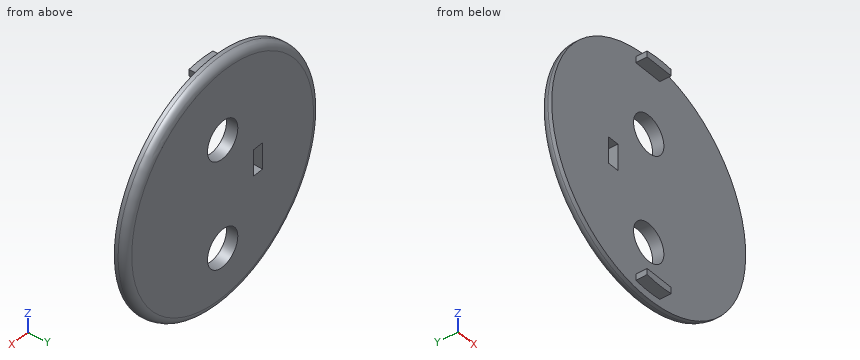
```python
from build123d import *

# Parameters (mm, degrees)
ESQUISSE2_R             = 32
ESQUISSE2_R_2           = 5
BOSS_EXTRU_1_DEPTH      = 3
CONG_1_R                = 2
BOSS_EXTRU_2_DEPTH      = 3
ESQUISSE4_W             = 3
ESQUISSE4_H             = 7
ENL_V_MAT_EXTRU_1_DEPTH = 10


with BuildPart() as part:
    # Esquisse2 → Boss.-Extru.1 (new body)
    with BuildSketch(Plane(origin=(0, 0, 0), x_dir=(1, 0, 0), z_dir=(0, 1, 0))):
        with Locations(Location((0, 0, 0), (0, 0, 270))):
            Circle(ESQUISSE2_R)
        with Locations(Location((0, -11.795669906, 0), (0, 0, 270))):
            Circle(ESQUISSE2_R_2, mode=Mode.SUBTRACT)
        with Locations(Location((0, 16.939646256, 0), (0, 0, 270))):
            Circle(ESQUISSE2_R_2, mode=Mode.SUBTRACT)
    extrude(amount=BOSS_EXTRU_1_DEPTH)

    # Congé1
    cong_1_edges = [part.edges().sort_by_distance(p)[0] for p in [
        (0, 3, -32),
    ]]
    fillet(cong_1_edges, radius=CONG_1_R)

    # Esquisse3 → Boss.-Extru.2 (add)
    with BuildSketch(Plane.XZ):
        with BuildLine():
            Line((-4.252814477, 29.697029633), (-4.252814477, 28.09287077))
            Line((-4.252814477, 28.09287077), (3.65484317, 28.09287077))
            Line((3.65484317, 28.09287077), (3.65484317, 29.776536424))
            add(Edge.make_bspline(
                [(-4.252814477, 29.697029633), (-0.301616898, 30.260197697), (3.65484317, 29.776536424)],
                knots=[0, 0, 0, 1, 1, 1], degree=2))
        make_face()
        with BuildLine():
            Line((-4.252814477, -28.09287077), (3.65484317, -28.09287077))
            Line((3.65484317, -28.09287077), (3.65484317, -29.776536424))
            add(Edge.make_bspline(
                [(-4.252814477, -29.697029633), (-0.301616898, -30.260197697), (3.65484317, -29.776536424)],
                knots=[0, 0, 0, 1, 1, 1], degree=2))
            Line((-4.252814477, -29.697029633), (-4.252814477, -28.09287077))
        make_face()
    extrude(amount=BOSS_EXTRU_2_DEPTH)

    # Esquisse4 → Enlèv. mat.-Extru.1 (cut)
    with BuildSketch(Plane(origin=(0, 3, 0), x_dir=(1, 0, 0), z_dir=(0, 1, 0))):
        with Locations((-11.703666828, 0.799999388)):
            Rectangle(ESQUISSE4_W, ESQUISSE4_H)
    extrude(amount=-ENL_V_MAT_EXTRU_1_DEPTH, mode=Mode.SUBTRACT)


solid = part.part
```
The listing builds one solid part. Answer for the finished solid, in the listing's coordinates (mm). Give positions to 0.01 mm unless a question says otherwise; leave off trailing zeros. Loops run counter-clockwise (first coordinate to the right, second up) from the corner with the lowest first, then second, coordinate; pieces in that order, holes last. Notation, with made-up numbers: (49.25, 85) - (83.25, 85) arc R17 ccw to (83.25, 109) - close; hole circle Ø2 at (-10, 11.5). An arc over 180 degrees is marked (long way). Answer as CSV lines item,"result". Start each with the question number.
Item 1: A cutting plane is placed at B-B on x = 0. Count the separate pieces of the cut face and the enclosed holes in it, then the cut area to 3 significant figures.
Item 2: A cutting plane is placed at A-A on z = 0. Determine the outline of the cut face in (x, y).
Item 3: Each of these flat-tipped pins is pushed along its axis until it touches: pin 1 (1.5 mm diameter, centred on y = 1, z = -2.5, fed in from +X); pin 2 (16 mm diameter, centred on x = 0, z = 11.8, fed in from -Y); pin 3 (0.8 mm diameter, centred on y = -1, z = -29, fed in from -X); pin 4 (3.5 mm diameter, centred on x = -1, y = -1, fed in from +Z). Where does it stop, or does it pass through?
Item 4: Find the intervals of material crossed by line 1 (Z direction, x = 3, y = 2); line 2 (Z direction, x = 0.5, y = 1.5); line 3 (Y direction, x = -23.5, z = -7), in increasing order. Write a range as from..to.
Found:
1,separate pieces,"3"
1,enclosed holes,"0"
1,area,"142 mm^2"
2,outline,"(-32, 0) - (-13.2, 0) - (-13.2, 3) - (-30, 3) arc R2 ccw to (-32, 1) - close; (-10.2, 0) - (32, 0) - (32, 1) arc R2 ccw to (30, 3) - (-10.2, 3) - close"
3,pin 1,"stops at x = 31.95"
3,pin 2,"stops at y = 0"
3,pin 3,"stops at x = -4.25"
3,pin 4,"stops at z = 32"
4,line 1,"z = -31.59..-20.94, -12.94..7.8, 15.8..31.59"
4,line 2,"z = -31.93..-21.91, -11.96..6.82, 16.77..31.93"
4,line 3,"y = 0..3"
